CAD build for the part. Positions are in the model's coordinates, mm. Face numbers are marked on the shaded views. Give positions to 0.01 mm unless a question says otherwise; leave off trailing zeros. Write each loop counter-clockwise with the first axis right and the second up, starting at its lowest first coordinate (ties: lowest second). Pieces come first, ordered by that corner, then holes. Notation, with made-up numbers: (-35.5, 22) - (21.5, 22) arc R27 cw to (21.5, 53) - close; hole circle Ø3 at (42.25, -31.75). An arc over 180 degrees is marked (long way). Answer as a JSON object with one key per item and string values.
from build123d import *

# Parameters (mm, degrees)
F1_DEPTH = 6.35


with BuildPart() as f1:
    # F0 (on Top) → F1 (new body)
    with BuildSketch(Plane.XY):
        with BuildLine():
            add(Edge.make_bspline(
                [(0, 71.2421610951), (-1.8717980289, 68.832793782), (-5.9054940485, 63.7394567312), (-10.2932083579, 53.2239591481), (-10.7742816294, 50.7587112719)],
                knots=[0, 0, 0, 0, 0.3881776272, 0.8302867615, 0.8302867615, 0.8302867615, 0.8302867615], degree=3))
            ThreePointArc((-10.7742816294, 50.7587112719), (-12.151414509, 45.5150408691), (-11.4572210078, 40.1381765744))
            add(Edge.make_bspline(
                [(-11.3991048065, 20.7600555156), (-11.7325351971, 22.9101453469), (-12.7530584769, 27.8294481961), (-11.8366984864, 35.6693833545), (-11.4572210078, 40.1381765744)],
                knots=[0, 0, 0, 0, 0.426568444, 1, 1, 1, 1], degree=3))
            Line((-11.3991048065, 20.7600555156), (-12.216145647, 16.6687367736))
            Line((-12.216145647, 16.6687367736), (-20.5436223185, 2.2451240799))
            Line((-20.5436223185, 2.2451240799), (-8.3274766714, -18.9138608535))
            Line((-8.3274766714, -18.9138608535), (8.3274766714, -18.9138608535))
            Line((8.3274766714, -18.9138608535), (20.5436223185, 2.2451240799))
            Line((20.5436223185, 2.2451240799), (12.216145647, 16.6687367736))
            Line((12.216145647, 16.6687367736), (11.3991048065, 20.7600555156))
            add(Edge.make_bspline(
                [(11.3991048065, 20.7600555156), (11.7325351971, 22.9101453469), (12.7530584769, 27.8294481961), (11.8366984864, 35.6693833545), (11.4572210078, 40.1381765744)],
                knots=[0, 0, 0, 0, 0.426568444, 1, 1, 1, 1], degree=3))
            ThreePointArc((11.4572210078, 40.1381765744), (12.151414509, 45.5150408691), (10.7742816294, 50.7587112719))
            add(Edge.make_bspline(
                [(0, 71.2421610951), (1.8717980289, 68.832793782), (5.9054940485, 63.7394567312), (10.2932083579, 53.2239591481), (10.7742816294, 50.7587112719)],
                knots=[0, 0, 0, 0, 0.3881776272, 0.8302867615, 0.8302867615, 0.8302867615, 0.8302867615], degree=3))
        make_face()
        with BuildLine():
            Line((-20.5436223185, 2.2451240799), (-12.216145647, 16.6687367736))
            Line((-12.216145647, 16.6687367736), (-13.2953060188, 16.6687367736))
            ThreePointArc((-13.2953060188, 16.6687367736), (-13.4997773753, 20.2820878122), (-14.7402806158, 23.6819798654))
            ThreePointArc((-14.7402806158, 23.6819798654), (-27.7067627464, 15.7853712662), (-27.984043385, 0.6061353941))
            ThreePointArc((-27.984043385, 0.6061353941), (-24.3555326782, 1.1738561923), (-21.1061885939, 2.885627169))
            Line((-21.1061885939, 2.885627169), (-20.5436223185, 2.2451240799))
        make_face()
        with BuildLine():
            Line((-8.3274766714, -18.9138608535), (-20.5436223185, 2.2451240799))
            Line((-20.5436223185, 2.2451240799), (-23.6782878637, -0.508113415))
            add(Edge.make_bspline(
                [(-23.6782878637, -0.508113415), (-25.7070354734, -1.294399142), (-30.4775383496, -2.8702514812), (-36.8089413655, -7.5838100911), (-40.4892910789, -10.1468438377)],
                knots=[0, 0, 0, 0, 0.426568444, 1, 1, 1, 1], degree=3))
            ThreePointArc((-40.4892910789, -10.1468438377), (-45.4928889014, -12.2340867779), (-49.3454742395, -16.0485540373))
            add(Edge.make_bspline(
                [(-61.6975213289, -35.6210805476), (-60.5468470431, -32.7953722472), (-58.1527357769, -26.7554204977), (-51.2399048911, -17.6977996497), (-49.3454742395, -16.0485540373)],
                knots=[0, 0, 0, 0, 0.3881776272, 0.8302867615, 0.8302867615, 0.8302867615, 0.8302867615], degree=3))
            add(Edge.make_bspline(
                [(-61.6975213289, -35.6210805476), (-58.6750490142, -36.0374215348), (-52.2472417284, -36.9840362335), (-40.9466965333, -35.5261594984), (-38.5711926101, -34.7101572345)],
                knots=[0, 0, 0, 0, 0.3881776272, 0.8302867615, 0.8302867615, 0.8302867615, 0.8302867615], degree=3))
            ThreePointArc((-38.5711926101, -34.7101572345), (-33.3414743924, -33.2809540912), (-29.0320700711, -29.9913327367))
            add(Edge.make_bspline(
                [(-12.2791830572, -20.2519421006), (-13.9745002763, -21.6157462049), (-17.7244798727, -24.959196715), (-24.9722428792, -28.0855732634), (-29.0320700711, -29.9913327367)],
                knots=[0, 0, 0, 0, 0.426568444, 1, 1, 1, 1], degree=3))
            Line((-12.2791830572, -20.2519421006), (-8.3274766714, -18.9138608535))
        make_face()
        with BuildLine():
            Line((8.3274766714, -18.9138608535), (-8.3274766714, -18.9138608535))
            Line((-8.3274766714, -18.9138608535), (-7.7878964856, -19.8484411502))
            ThreePointArc((-7.7878964856, -19.8484411502), (-10.8149145995, -21.8321940585), (-13.1390558675, -24.6064474049))
            ThreePointArc((-13.1390558675, -24.6064474049), (0.1828488485, -31.8874460281), (13.4670930431, -24.5379601691))
            ThreePointArc((13.4670930431, -24.5379601691), (11.1611770562, -21.6794381182), (8.0540678628, -19.7213090839))
            Line((8.0540678628, -19.7213090839), (8.3274766714, -18.9138608535))
        make_face()
        with BuildLine():
            Line((20.5436223185, 2.2451240799), (8.3274766714, -18.9138608535))
            Line((8.3274766714, -18.9138608535), (12.2791830572, -20.2519421006))
            add(Edge.make_bspline(
                [(12.2791830572, -20.2519421006), (13.9745002763, -21.6157462049), (17.7244798727, -24.959196715), (24.9722428792, -28.0855732634), (29.0320700711, -29.9913327367)],
                knots=[0, 0, 0, 0, 0.426568444, 1, 1, 1, 1], degree=3))
            ThreePointArc((29.0320700711, -29.9913327367), (33.3414743924, -33.2809540912), (38.5711926101, -34.7101572345))
            add(Edge.make_bspline(
                [(61.6975213289, -35.6210805476), (58.6750490142, -36.0374215348), (52.2472417284, -36.9840362335), (40.9466965333, -35.5261594984), (38.5711926101, -34.7101572345)],
                knots=[0, 0, 0, 0, 0.3881776272, 0.8302867615, 0.8302867615, 0.8302867615, 0.8302867615], degree=3))
            add(Edge.make_bspline(
                [(61.6975213289, -35.6210805476), (60.5468470431, -32.7953722472), (58.1527357769, -26.7554204977), (51.2399048911, -17.6977996497), (49.3454742395, -16.0485540373)],
                knots=[0, 0, 0, 0, 0.3881776272, 0.8302867615, 0.8302867615, 0.8302867615, 0.8302867615], degree=3))
            ThreePointArc((49.3454742395, -16.0485540373), (45.4928889014, -12.2340867779), (40.4892910789, -10.1468438377))
            add(Edge.make_bspline(
                [(23.6782878637, -0.508113415), (25.7070354734, -1.294399142), (30.4775383496, -2.8702514812), (36.8089413655, -7.5838100911), (40.4892910789, -10.1468438377)],
                knots=[0, 0, 0, 0, 0.426568444, 1, 1, 1, 1], degree=3))
            Line((23.6782878637, -0.508113415), (20.5436223185, 2.2451240799))
        make_face()
        with BuildLine():
            Line((13.0521207311, 16.8356819149), (12.216145647, 16.6687367736))
            Line((12.216145647, 16.6687367736), (20.5436223185, 2.2451240799))
            Line((20.5436223185, 2.2451240799), (21.0832025044, 3.1797043765))
            ThreePointArc((21.0832025044, 3.1797043765), (24.3146919748, 1.5501062464), (27.8793364832, 0.9244675395))
            ThreePointArc((27.8793364832, 0.9244675395), (27.5239138979, 16.1020747619), (14.516950342, 23.931824775))
            ThreePointArc((14.516950342, 23.931824775), (13.194355622, 20.5055819259), (13.0521207311, 16.8356819149))
        make_face()
    extrude(amount=F1_DEPTH)


solid = f1.part
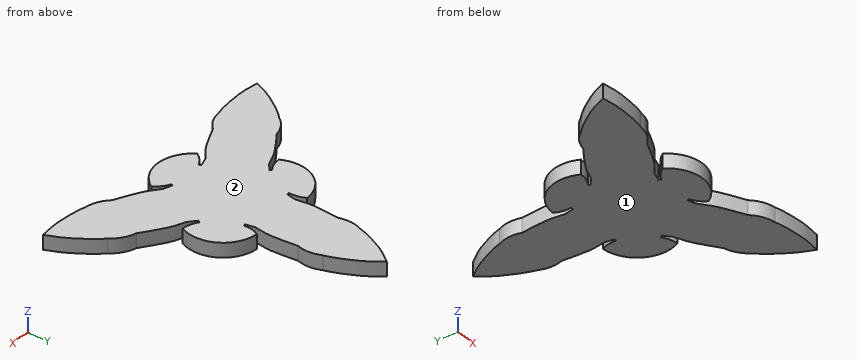
(1) Flat gauge pins, fed straight in: P1, Ø1.5, axis at y = 56.5, z = 5, coming from the +X side; P2, Ø1.5, axis at x = 36.5, z = 2, coming from the -Y side; P3, Ø1, axis at y = 53, z = 5, coming from the +X side. Where does each tip first touch, or does it go through?
Answer key:
{"P1": "stops at x = 9.1", "P2": "stops at y = -34.55", "P3": "stops at x = 10.3"}
(2) Saw through at A-A, the plane y = 10. Give the cut face in (x, z), and give its area (3 significant figures).
Answer key:
{"outline": "(-29.66, 0) - (29.55, 0) - (29.55, 6.35) - (-29.66, 6.35) - close", "area": "376 mm²"}
(3) Probe L1, parallel to X at y = -28.5, z = 3; L2, parallel to X at y = 44.5, z = 1.5; L3, parallel to X at y = -27, z = 0.75. List the from-to ranges inside material, lowest first. Write a range as [from, to].
Answer key:
{"L1": "x = [-58.47, -25.81], [-9.62, 9.9], [25.81, 58.47]", "L2": "x = [-12.18, 12.18]", "L3": "x = [-57.63, -22.62], [-11.26, 11.55], [22.62, 57.63]"}
(4) Pull direction Z, two halves, no side cores. Call the marked faces 1 and 2: pulls with the +Z half, pulls with the -Z half, needs draft (parallel to the pull), parting line crosses it, or undercut.
Answer key:
{"face 1": "pulls with the -Z half", "face 2": "pulls with the +Z half"}
